Geometry check sheet. Reference: the model listing, model coordinates, mm. Face numbers are marked on the shaded views. A direction names the side the tool comes from. Round coordinates to 2 decimals unless told otherwise and drop trailing zeros. Write each loop counter-clockwise with the first axis right and the second up, starting at its lowest first coordinate (ties: lowest second). Pieces come first, ordered by that corner, then holes.
Item 1: Scan lines: probe 1 along X at (y, z) = (33, -78); probe 2 along Y at (x, z) = (34, -29); probe 3 along Z at (x, y) = (21, 39.5). Record each from-to range of solid material in increasing order.
Item 2: Cross-section at A-A (z = -62). Enter the section's corners in (x, y).
Item 3: Access from +Z, -Z, +X, -X, +Y, -Y to the whole of each face (thin tool, end or side, straight path). Record for the marked faces 1, 2 and 3.
Item 4: Depth check by flat-ended pin: P1, Ø1.5, axis at y = 35, z = 5.5, coming from the -X side; P2, Ø7.5, axis at y = 44.5, z = -78, coming from the +X side; P3, Ø15, axis at x = 20.5, y = 22.5, coming from the +Z side. Enter the tip coordinate at first touch or a pass-through.
Item 5: Cross-section at B-B (x = 74). Enter the section's corners in (y, z), then the cut area to 3 significant figures.
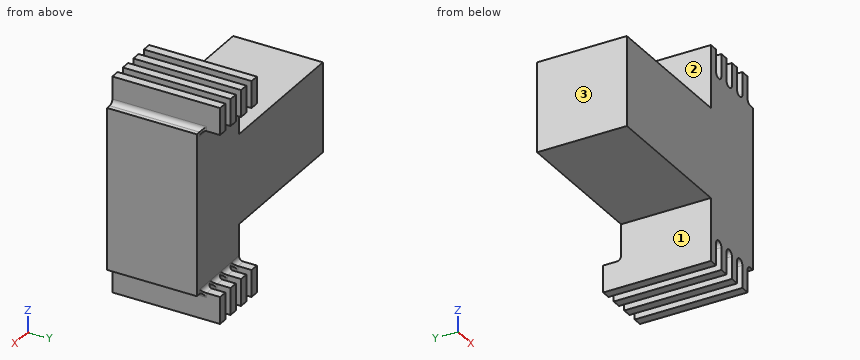
from build123d import *

# Parameters (mm, degrees)
BOSS_EXTRUDE1_DEPTH             = 50
SKETCH2_W                       = 5
SKETCH2_H                       = 15
BOSS_EXTRUDE2_DEPTH             = 10
BOSS_EXTRUDE2_DIRECTION_2_REACH = 149.648
FILLET1_R                       = 2.5
FILLET2_R                       = 2.5
FILLET4_R                       = 2.5


with BuildPart() as part:
    # Sketch1 → Boss-Extrude1 (new body)
    with BuildSketch(Plane(origin=(0, 0, 0), x_dir=(1, 0, 0), z_dir=(0, 1, 0))):
        Polygon((80, 50), (80, 70), (120, 70), (120, -20), (80, -20), (80, 0), (0, 0), (0, 50), align=None)
    extrude(amount=BOSS_EXTRUDE1_DEPTH)

    # Sketch2 → Boss-Extrude2 (add)
    with BuildSketch(Plane(origin=(0, 50, 0), x_dir=(1, 0, 0), z_dir=(0, 1, 0))):
        with Locations((82.5, -27.5)):
            Rectangle(SKETCH2_W, SKETCH2_H)
        with Locations((92.5, -27.5)):
            Rectangle(SKETCH2_W, SKETCH2_H)
        with Locations((102.5, -27.5)):
            Rectangle(SKETCH2_W, SKETCH2_H)
        with Locations((112.5, -27.5)):
            Rectangle(SKETCH2_W, SKETCH2_H)
        with Locations((112.5, 77.5)):
            Rectangle(SKETCH2_W, SKETCH2_H)
        with Locations((102.5, 77.5)):
            Rectangle(SKETCH2_W, SKETCH2_H)
        with Locations((92.5, 77.5)):
            Rectangle(SKETCH2_W, SKETCH2_H)
        with Locations((82.5, 77.5)):
            Rectangle(SKETCH2_W, SKETCH2_H)
    extrude(amount=BOSS_EXTRUDE2_DEPTH)

    # Boss-Extrude2 direction 2: up to this face of the body (flat: up to its plane)
    boss_extrude2_direction_2_end = Plane(part.part.faces().sort_by_distance((68.421052632, 0, -25))[0])
    # Sketch2 → Boss-Extrude2 direction 2 (add, up to the picked face)
    with BuildSketch(Plane(origin=(0, 50, 0), x_dir=(1, 0, 0), z_dir=(0, 1, 0)), mode=Mode.PRIVATE) as boss_extrude2_direction_2_sk1:
        with Locations((82.5, -27.5)):
            Rectangle(SKETCH2_W, SKETCH2_H)
    boss_extrude2_direction_2_tool1 = split(extrude(boss_extrude2_direction_2_sk1.sketch, amount=-BOSS_EXTRUDE2_DIRECTION_2_REACH, mode=Mode.PRIVATE), bisect_by=boss_extrude2_direction_2_end, keep=Keep.BOTH, mode=Mode.PRIVATE)
    # Sketch2 → Boss-Extrude2 direction 2 (add, up to the picked face)
    with BuildSketch(Plane(origin=(0, 50, 0), x_dir=(1, 0, 0), z_dir=(0, 1, 0)), mode=Mode.PRIVATE) as boss_extrude2_direction_2_sk2:
        with Locations((92.5, -27.5)):
            Rectangle(SKETCH2_W, SKETCH2_H)
    boss_extrude2_direction_2_tool2 = split(extrude(boss_extrude2_direction_2_sk2.sketch, amount=-BOSS_EXTRUDE2_DIRECTION_2_REACH, mode=Mode.PRIVATE), bisect_by=boss_extrude2_direction_2_end, keep=Keep.BOTH, mode=Mode.PRIVATE)
    # Sketch2 → Boss-Extrude2 direction 2 (add, up to the picked face)
    with BuildSketch(Plane(origin=(0, 50, 0), x_dir=(1, 0, 0), z_dir=(0, 1, 0)), mode=Mode.PRIVATE) as boss_extrude2_direction_2_sk3:
        with Locations((102.5, -27.5)):
            Rectangle(SKETCH2_W, SKETCH2_H)
    boss_extrude2_direction_2_tool3 = split(extrude(boss_extrude2_direction_2_sk3.sketch, amount=-BOSS_EXTRUDE2_DIRECTION_2_REACH, mode=Mode.PRIVATE), bisect_by=boss_extrude2_direction_2_end, keep=Keep.BOTH, mode=Mode.PRIVATE)
    # Sketch2 → Boss-Extrude2 direction 2 (add, up to the picked face)
    with BuildSketch(Plane(origin=(0, 50, 0), x_dir=(1, 0, 0), z_dir=(0, 1, 0)), mode=Mode.PRIVATE) as boss_extrude2_direction_2_sk4:
        with Locations((112.5, -27.5)):
            Rectangle(SKETCH2_W, SKETCH2_H)
    boss_extrude2_direction_2_tool4 = split(extrude(boss_extrude2_direction_2_sk4.sketch, amount=-BOSS_EXTRUDE2_DIRECTION_2_REACH, mode=Mode.PRIVATE), bisect_by=boss_extrude2_direction_2_end, keep=Keep.BOTH, mode=Mode.PRIVATE)
    # Sketch2 → Boss-Extrude2 direction 2 (add, up to the picked face)
    with BuildSketch(Plane(origin=(0, 50, 0), x_dir=(1, 0, 0), z_dir=(0, 1, 0)), mode=Mode.PRIVATE) as boss_extrude2_direction_2_sk5:
        with Locations((112.5, 77.5)):
            Rectangle(SKETCH2_W, SKETCH2_H)
    boss_extrude2_direction_2_tool5 = split(extrude(boss_extrude2_direction_2_sk5.sketch, amount=-BOSS_EXTRUDE2_DIRECTION_2_REACH, mode=Mode.PRIVATE), bisect_by=boss_extrude2_direction_2_end, keep=Keep.BOTH, mode=Mode.PRIVATE)
    # Sketch2 → Boss-Extrude2 direction 2 (add, up to the picked face)
    with BuildSketch(Plane(origin=(0, 50, 0), x_dir=(1, 0, 0), z_dir=(0, 1, 0)), mode=Mode.PRIVATE) as boss_extrude2_direction_2_sk6:
        with Locations((102.5, 77.5)):
            Rectangle(SKETCH2_W, SKETCH2_H)
    boss_extrude2_direction_2_tool6 = split(extrude(boss_extrude2_direction_2_sk6.sketch, amount=-BOSS_EXTRUDE2_DIRECTION_2_REACH, mode=Mode.PRIVATE), bisect_by=boss_extrude2_direction_2_end, keep=Keep.BOTH, mode=Mode.PRIVATE)
    # Sketch2 → Boss-Extrude2 direction 2 (add, up to the picked face)
    with BuildSketch(Plane(origin=(0, 50, 0), x_dir=(1, 0, 0), z_dir=(0, 1, 0)), mode=Mode.PRIVATE) as boss_extrude2_direction_2_sk7:
        with Locations((92.5, 77.5)):
            Rectangle(SKETCH2_W, SKETCH2_H)
    boss_extrude2_direction_2_tool7 = split(extrude(boss_extrude2_direction_2_sk7.sketch, amount=-BOSS_EXTRUDE2_DIRECTION_2_REACH, mode=Mode.PRIVATE), bisect_by=boss_extrude2_direction_2_end, keep=Keep.BOTH, mode=Mode.PRIVATE)
    # Sketch2 → Boss-Extrude2 direction 2 (add, up to the picked face)
    with BuildSketch(Plane(origin=(0, 50, 0), x_dir=(1, 0, 0), z_dir=(0, 1, 0)), mode=Mode.PRIVATE) as boss_extrude2_direction_2_sk8:
        with Locations((82.5, 77.5)):
            Rectangle(SKETCH2_W, SKETCH2_H)
    boss_extrude2_direction_2_tool8 = split(extrude(boss_extrude2_direction_2_sk8.sketch, amount=-BOSS_EXTRUDE2_DIRECTION_2_REACH, mode=Mode.PRIVATE), bisect_by=boss_extrude2_direction_2_end, keep=Keep.BOTH, mode=Mode.PRIVATE)
    add(boss_extrude2_direction_2_tool1.solids().sort_by(Axis((82.5, 50, 27.5), (0, -1, 0)))[0])
    add(boss_extrude2_direction_2_tool2.solids().sort_by(Axis((92.5, 50, 27.5), (0, -1, 0)))[0])
    add(boss_extrude2_direction_2_tool3.solids().sort_by(Axis((102.5, 50, 27.5), (0, -1, 0)))[0])
    add(boss_extrude2_direction_2_tool4.solids().sort_by(Axis((112.5, 50, 27.5), (0, -1, 0)))[0])
    add(boss_extrude2_direction_2_tool5.solids().sort_by(Axis((112.5, 50, -77.5), (0, -1, 0)))[0])
    add(boss_extrude2_direction_2_tool6.solids().sort_by(Axis((102.5, 50, -77.5), (0, -1, 0)))[0])
    add(boss_extrude2_direction_2_tool7.solids().sort_by(Axis((92.5, 50, -77.5), (0, -1, 0)))[0])
    add(boss_extrude2_direction_2_tool8.solids().sort_by(Axis((82.5, 50, -77.5), (0, -1, 0)))[0])

    # Fillet1
    fillet1_edges = [part.edges().sort_by_distance(p)[0] for p in [
        (85, 25, -70),
        (85, 25, 20),
        (115, 25, -70),
        (110, 25, -70),
        (95, 25, 20),
        (90, 25, 20),
        (105, 25, 20),
        (100, 25, 20),
        (115, 25, 20),
        (110, 25, 20),
        (105, 25, -70),
        (100, 25, -70),
        (95, 25, -70),
        (90, 25, -70),
    ]]
    fillet(fillet1_edges, radius=FILLET1_R - 0.0001)  # a hair under: the kernel refuses the full size

    # Fillet2
    fillet2_edges = [part.edges().sort_by_distance(p)[0] for p in [
        (82.5, 50, -70),
        (82.5, 50, 20),
        (112.5, 50, -70),
        (92.5, 50, 20),
        (102.5, 50, 20),
        (112.5, 50, 20),
        (102.5, 50, -70),
        (92.5, 50, -70),
    ]]
    fillet(fillet2_edges, radius=FILLET2_R)

    # Fillet4
    fillet4_edges = [part.edges().sort_by_distance(p)[0] for p in [
        (110, 50, -69.99995),
        (100, 50, -69.99995),
        (90, 50, -69.99995),
        (110, 50, 19.99995),
        (100, 50, 19.99995),
        (90, 50, 19.99995),
        (115, 50, -69.99995),
        (105, 50, -69.99995),
        (95, 50, -69.99995),
        (85, 50, -69.99995),
        (85, 50, 19.99995),
        (95, 50, 19.99995),
        (105, 50, 19.99995),
        (115, 50, 19.99995),
    ]]
    fillet(fillet4_edges, radius=FILLET4_R - 0.0001)  # a hair under: the kernel refuses the full size


solid = part.part
Resolved:
1. probe 1: x = 80 to 85, 90 to 95, 100 to 105, 110 to 115
1. probe 2: y = 0 to 50
1. probe 3: z = -50 to 0
2. outline: (80, 0) - (120, 0) - (120, 50) - (80, 50) - close
3. face 1: -Z, -X, +Y, -Y
3. face 2: +Z, -X, +Y, -Y
3. face 3: +Z, -Z, -X, +Y, -Y
4. P1: stops at x = 80
4. P2: stops at x = 115
4. P3: stops at z = 0
5. outline: (0, -50) - (50, -50) - (50, 0) - (0, 0) - close
5. area: 2,500 mm2
